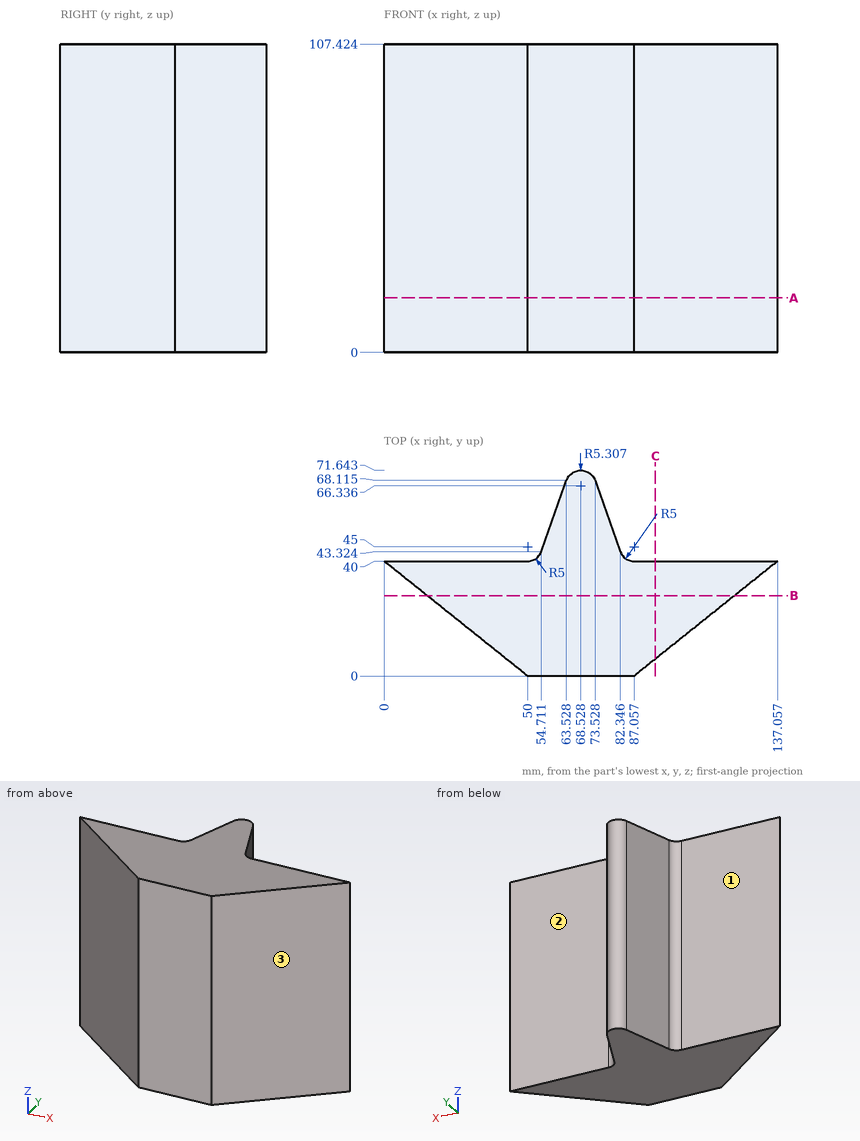
Can you work these out from the drawing? Everything is in mm from the part's minimum corner. A direction names the side the tool comes from. Coordinates: 2 decimals unless noted, no trailing zeros. Loops run counter-clockwise (first coordinate to the right, second up) from the corner with the lowest first, then second, coordinate; pieces in that order, holes last. Notation, with made-up numbers: M 7.5,-1 L 24.5,-1 A28 cw 24.5,23 Z; hole C 44,68 d3. An arc over 180 degrees is marked long. Put each result on its own line as item: value. Start each with the question number.
(1) Suppose I cut it at C-C on x = 94.5. Please give me the cut outline in (y, z) (1 decimal), then the cut area to 3 significant figures.
(2) Suppose I cut it at A-A on z = 19. Please give me the cut outline in (x, y) (1 decimal), then the cut area to 4 significant figures.
(3) For the marked faces 1, 2 and 3, which set-ups out of +Z, -Z, +X, -X, +Y, -Y let a thin tool reach every point of the face, with its end or its side?
(4) I need wall thicknesses on line 1 (Y direction, x = 86, z = 92); line 2 (Y direction, x = 96, z = 58) (1 decimal); line 3 (X direction, y = 44.5, z = 69). Which ranges of each line are inside material? Lowest first, please. Write a range as from..to.
(5) Will these pins go through, and if not, where does the flat tip stop? P1, Ø2, axis at y = 31.5, z = 20.5, coming from the -X side (1 decimal); P2, Ø5, axis at x = 21, y = 20.5, coming from the -Z side; P3, Ø5, axis at y = 16, z = 75, coming from the -X side (1 decimal); P4, Ø4, axis at x = 91.5, z = 71, coming from the +Y side.
(6) Suppose I cut it at B-B on y = 28. Please give me the cut outline in (x, z), then the cut area to 3 significant figures.
Solutions:
1. outline: M 6,0 L 40,0 L 40,107.4 L 6,107.4 Z
1. area: 3,660 mm2
2. outline: M 0,40 L 50,0 L 87.1,0 L 137.1,40 L 87.1,40 A5 cw 82.3,43.3 L 73.5,68.1 A5.3 ccw 63.5,68.1 L 54.7,43.3 A5 cw 50,40 Z
2. area: 4,075 mm2
3. face 1: +Z, -Z, -X, +Y
3. face 2: +Z, -Z, +X, +Y
3. face 3: +Z, -Z, +X, -Y
4. line 1: y = 0..40.11
4. line 2: y = 7.2..40
4. line 3: x = 55.13..81.93
5. P1: stops at x = 9.4
5. P2: stops at z = 0
5. P3: stops at x = 26.9
5. P4: stops at y = 40
6. outline: M 15,0 L 122.06,0 L 122.06,107.42 L 15,107.42 Z
6. area: 11,500 mm2
